```python
from build123d import *

# Parameters (mm, degrees)
SKETCH_2_R          = 0.65
EXTRUDE_1_DEPTH     = 33
CUT_EXTRUDE_START   = -6.4
SKETCH_3_R          = 0.65
SKETCH_3_R_2        = 0.45
CUT_EXTRUDE_2_DEPTH = 6.4
SKETCH_5_R          = 1.65
EXTRUDE_2_DEPTH     = 2


with BuildPart() as part:
    # 草图2 → 凸台-拉伸1 (new body)
    with BuildSketch(Plane(origin=(0, 0, 0), x_dir=(1, 0, 0), z_dir=(0, 1, 0))):
        with Locations(Location((0, 0, 0), (0, 0, 270))):
            Circle(SKETCH_2_R)
    extrude(amount=EXTRUDE_1_DEPTH)

    # 草图3 → 切除-拉伸2 (cut)
    with BuildSketch(Plane(origin=(0, 33, 0), x_dir=(1, 0, 0), z_dir=(0, 1, 0)).offset(CUT_EXTRUDE_START)):
        with Locations(Location((0, 0, 0), (0, 0, 270))):
            Circle(SKETCH_3_R)
        with Locations(Location((0, 0, 0), (0, 0, 270))):
            Circle(SKETCH_3_R_2, mode=Mode.SUBTRACT)
    extrude(amount=CUT_EXTRUDE_2_DEPTH, mode=Mode.SUBTRACT)

    # 草图5 → 凸台-拉伸2 (add)
    with BuildSketch(Plane(origin=(0, 33, 0), x_dir=(1, 0, 0), z_dir=(0, 1, 0))):
        with Locations(Location((0, 0, 0), (0, 0, 270))):
            Circle(SKETCH_5_R)
    extrude(amount=EXTRUDE_2_DEPTH)


solid = part.part
```
Read the model definition and answer for the solid it produces. Units are mm, in the model's axes. A direction names the side the tool comes from. Coordinates: 2 decimals unless noted, no trailing zeros. Loops run counter-clockwise (first coordinate to the right, second up) from the corner with the lowest first, then second, coordinate; pieces in that order, holes last.
(1) Consider line 1 along Y through (x, z) = (-0.8, 0); line 2 along Y through (x, z) = (0.05, 0.6); line 3 along X through (y, z) = (3, 0.1). Determine where each line is inside the solid, lowest interval first.
Solution:
line 1: y = 33 to 35
line 2: y = 0 to 26.6, 33 to 35
line 3: x = -0.64 to 0.64
(2) The part is cut by section D-D (y = 27). Determine the outline of the cut face in (x, z).
Solution:
outline: circle Ø0.9 at (0, 0)
(3) The part is cut by section B-B (x = 0). Determine the outline of the cut face in (y, z).
Solution:
outline: (0, -0.65) - (26.6, -0.65) - (26.6, -0.45) - (33, -0.45) - (33, -1.65) - (35, -1.65) - (35, 1.65) - (33, 1.65) - (33, 0.45) - (26.6, 0.45) - (26.6, 0.65) - (0, 0.65) - close
(4) The part is cut by section A-A (z = 0). Determine the outline of the cut face in (x, y), and give its area (3 significant figures).
Solution:
outline: (-1.65, 33) - (-0.45, 33) - (-0.45, 26.6) - (-0.65, 26.6) - (-0.65, 0) - (0.65, 0) - (0.65, 26.6) - (0.45, 26.6) - (0.45, 33) - (1.65, 33) - (1.65, 35) - (-1.65, 35) - close
area: 46.9 mm2
(5) The part is cut by section C-C (y = 15). Determine the outline of the cut face in (x, z).
Solution:
outline: circle Ø1.3 at (0, 0)
(6) A tool of negligible diameter and unlimited length cuts with its end or side. For faces 1 (the face through (0, 0, 0)), 2 (the face through (0.2, 13.11, 0.62)), 3 (the face through (-0.172, 29.755, 0.416)), from which of +Z, -Z, +X, -X, +Y, -Y can it reach the whole face along a straight path? Write none if from no direction.
Solution:
face 1: +Z, -Z, +X, -X, -Y
face 2: -Y
face 3: none
